```python
from build123d import *

# Parameters (mm, degrees)
BOSS_EXTRUDE1_DEPTH = 166.124


with BuildPart() as part:
    # Sketch1 → Boss-Extrude1 (new body)
    with BuildSketch(Plane(origin=(0, 0, 0), x_dir=(0, 0, -1), z_dir=(1, 0, 0))):
        with BuildLine():
            Line((1.31223354, 0), (30, 0))
            Line((30, 0), (30, 3.175))
            Line((30, 3.175), (42.665653227, 3.175))
            ThreePointArc((42.665653227, 3.175), (47.051803052, 0.575351996), (46.876974623, -4.520324118))
            Line((46.876974623, -4.520324118), (32.674189086, -26.711530815))
            Line((32.674189086, -26.711530815), (30, -25))
            Line((30, -25), (15.038789484, -48.376211248))
            ThreePointArc((15.038789484, -48.376211248), (14.046652384, -48.825851708), (13.232341269, -48.102380923))
            Line((13.232341269, -48.102380923), (0.348049605, -1.265234498))
            ThreePointArc((0.348049605, -1.265234498), (0.516861143, -0.393878931), (1.31223354, 0))
        make_face()
    extrude(amount=BOSS_EXTRUDE1_DEPTH)


solid = part.part
```
For this review, take the finished solid that the model builds, in its own axes (mm). A direction names the side the tool comes from. Round coordinates to 2 decimals unless told otherwise and drop trailing zeros. Write each loop counter-clockwise with the first axis right and the second up, starting at its lowest first coordinate (ties: lowest second). Pieces come first, ordered by that corner, then holes. Notation, with made-up numbers: M -1.5,72.25 L 40.5,72.25 A25 cw 40.5,96.25 Z; hole C 76,71 d2. An arc over 180 degrees is marked long. One line per item, written item: value. Start each with the question number.
(1) We need section A-A (x = 124.5). Give the boundary of the cut face in (y, z) (3 decimals).
(2) We need section B-B (z = -3.5). Give the boundary of the cut face in (x, y), and give its area (3 significant figures).
(3) We need section C-C (y = -39.5). Give the boundary of the cut face in (x, z), and give its area (3 significant figures).
(4) Wall thickness on line 1 (Z direction, x = 73, y = -26); line 2 (Y direction, x = 105, z = -40) (3 decimals); line 3 (Y direction, x = 140, z = -31) (3 decimals): over which ranges is each line inside the solid? List them lowest first.
(5) Insertion check: pin 1 (8 mm diameter, centred on x = 65.5, z = -35, fed in from -Y); pin 2 (8 mm diameter, centred on x = 37, y = -30, fed in from -Z); pin 3 (5 mm diameter, centred on x = 38.5, y = -8, fed in from +Z). Each pin has a flat end and moves straight along its axis. Give the tip position at first contact, or say it passes through.
(6) Machinability: for faces 1 (the flat face through (166.124, -17, -24)), 2 (the flat face through (82, 0, -15)), which of the approach directions +Z, -Z, +X, -X, +Y, -Y give a long, thin tool a straight path to every point of the face, cutting with its end or side? Answer none if there is none.
Result:
1. outline: M -48.376,-15.039 L -25,-30 L -26.712,-32.674 L -4.52,-46.877 A5 ccw 3.175,-42.666 L 3.175,-30 L 0,-30 L 0,-1.312 A1 ccw -1.265,-0.348 L -48.102,-13.232 A1 ccw Z
2. outline: M 0,-12.72 L 166.12,-12.72 L 166.12,0 L 0,0 Z
2. area: 2,110 mm²
3. outline: M 0,-20.72 L 166.12,-20.72 L 166.12,-10.87 L 0,-10.87 Z
3. area: 1,640 mm²
4. line 1: -33.13 to -31.56, -29.36 to -7.15
4. line 2: -15.265 to 3.175
4. line 3: -25.64 to 3.175
5. pin 1: y = -26.71
5. pin 2: z = -33.13
5. pin 3: z = -1.51
6. face 1: +Z, -Z, +X, +Y, -Y
6. face 2: +Z, +X, -X, +Y
